Autodesk Inventor part; units mm, degrees
ref_plane "YZ Plane" through (0, 0, 0) normal (1, 0, 0) x (0, 1, 0)
ref_plane "XZ Plane" through (0, 0, 0) normal (0, 1, 0) x (-1, 0, 0)
ref_plane "XY Plane" through (0, 0, 0) normal (0, 0, 1) x (1, 0, 0)
sketch "草图1" plane through (0, 0, 0) normal (0, 0, 1) x (1, 0, 0)
  circle A0 centre (9, 0) radius 2.5 construction
  circle A1 centre (0, 0) radius 2.5 construction
  circle A2 centre (0, 0) radius 2.5
  circle A3 centre (0, 0) radius 3.5
  line L0 (10.5, 3.5) -> (0, 3.5)
  line L1 (0, -3.5) -> (10.5, -3.5)
  circle A4 centre (10.5, 0) radius 2.5 construction
  circle A5 centre (10.5, 0) radius 2.5
  circle A6 centre (10.5, 0) radius 3.5
  line L2 (0, 0) -> (9.7373, 0) construction
  point P0 (1, 4.5)
  point P1 (1, -2.5)
  dimension "d4" = 7
  dimension "d7" = 7
  dimension "d8" = 10.5
  dimension "d9" = 10.5
extrude "拉伸1" add sketch "草图1" along normal mid plane 7.5
fillet "圆角1" radius 1 8 edges at (-3.5, 0, 3.75) (5.25, -3.5, 3.75) (14, 0, 3.75) (5.25, 3.5, 3.75) (14, 0, -3.75) (5.25, -3.5, -3.75) (-3.5, 0, -3.75) (5.25, 3.5, -3.75)
equation "\"d9\" = d8"
properties part number "链" material "ABS 塑料"
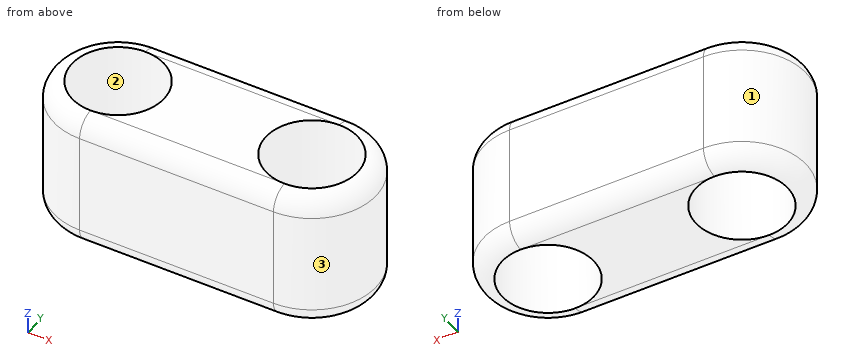
Input: part model. Units: mm. Frame: model coordinates. Face numbers are marked on the shaded views. Give positions to 0.01 mm unless a question says otherwise; leave off trailing zeros. Write each loop counter-clockwise with the first axis right and the second up, starting at its lowest first coordinate (ties: lowest second). Pieces come first, ordered by that corner, then holes. Notation, with made-up numbers: M 19.25,29 L 67.25,29 A5 ccw 67.25,36 Z; hole C 21,-22 d3. An arc over 180 degrees is marked long. Write item = value, one per line. Start each with the question number.
1) Draft query along X for the marked faces 1, 2 and 3. Return one class per face: +X half, -X half, draft (parallel to the pull), parting line (faces both ways), or undercut.
2) Cut plane D-D on x = 1. Return the cut outline in (y, z).
3) Cut plane B-B on z = -0.75. Return the cut outline in (x, y), then the cut area to 3 significant figures.
4) Cut plane C-C on y = 0. Count the separate pieces of the cut face and the enclosed holes in it, then the cut area to 3 significant figures.
5) Material intervals for line 1 along Y through (x, z) = (10.5, -0.25); line 2 along X through (y, z) = (0.25, 2.25); line 3 along X through (y, z) = (0.5, 3), sorted ascending. Write a range as [from, to].
6) First-contact query: pin 1 Ø3 at (y, z) = (0.5, -1) entering from -X; pin 2 Ø1 at (y, z) = (2.5, 0) entering from +X. Flat tips, straight axial feed; report the tip coordinate or a pass-through.
7) Cut plane A-A on x = 7.75. Return the cut outline in (y, z).
Solved:
q1.face_1 = -X half
q1.face_2 = undercut
q1.face_3 = +X half
q2.outline = M -3.5,-2.75 A1 ccw -2.5,-3.75 L -2.29,-3.75 L -2.29,3.75 L -2.5,3.75 A1 ccw -3.5,2.75 Z; M 2.29,-3.75 L 2.5,-3.75 A1 ccw 3.5,-2.75 L 3.5,2.75 A1 ccw 2.5,3.75 L 2.29,3.75 Z
q3.outline = M 0,-3.5 L 10.5,-3.5 A3.5 ccw 10.5,3.5 L 0,3.5 A3.5 ccw Z; hole C 0,0 d5; hole C 10.5,0 d5
q3.area = 72.7 mm2
q4.separate_pieces = 3
q4.enclosed_holes = 0
q4.area = 55.4 mm2
q5.line_1 = [-3.5, -2.5], [2.5, 3.5]
q5.line_2 = [-3.49, -2.49], [2.49, 8.01], [12.99, 13.99]
q5.line_3 = [-3.43, -2.45], [2.45, 8.05], [12.95, 13.93]
q6.pin_1 = -3.5
q6.pin_2 = 13.37
q7.outline = M -3.5,-2.75 A1 ccw -2.5,-3.75 L 2.5,-3.75 A1 ccw 3.5,-2.75 L 3.5,2.75 A1 ccw 2.5,3.75 L -2.5,3.75 A1 ccw -3.5,2.75 Z
